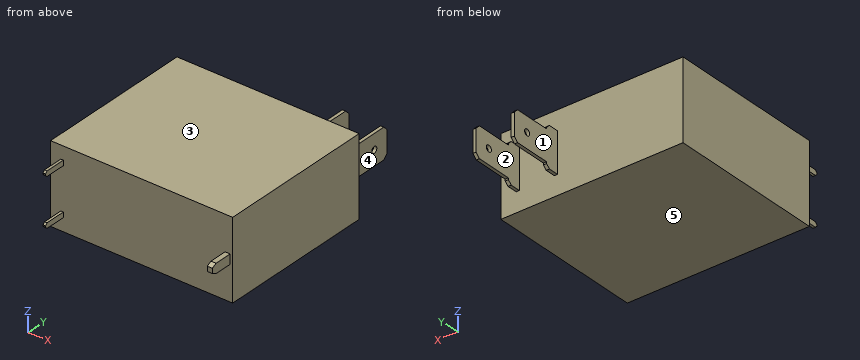
from build123d import *

# Parameters (mm, degrees)
CROQUIS1_W              = 28.6
CROQUIS1_H              = 12.4
SALIENTE_EXTRUIR1_DEPTH = 24.9
CROQUIS2_R              = 0.5
SALIENTE_EXTRUIR2_DEPTH = 0.25
SALIENTE_EXTRUIR3_DEPTH = 0.4
SALIENTE_EXTRUIR4_DEPTH = 0.2


with BuildPart() as part:
    # Croquis1 → Saliente-Extruir1 (new body)
    with BuildSketch(Plane(origin=(0, 0, 0), x_dir=(1, 0, 0), z_dir=(0, 1, 0))):
        with Locations((14.3, 6.2)):
            Rectangle(CROQUIS1_W, CROQUIS1_H)
    extrude(amount=SALIENTE_EXTRUIR1_DEPTH)

    # Croquis2 → Saliente-Extruir2 (add, symmetric)
    with BuildSketch(Plane(origin=(25.95, 0, 0), x_dir=(0, 0, -1), z_dir=(1, 0, 0))):
        Polygon((3.05, 24.9), (3.05, 26.504259841), (3.5733005, 27.05), (3.825, 27.05), (3.825, 32.761976859), (4.463023141, 33.4), (7.936976859, 33.4), (8.575, 32.761976859), (8.575, 27.05), (8.8266995, 27.05), (9.35, 26.504259841), (9.35, 24.9), align=None)
        with Locations((6.2, 30.9)):
            Circle(CROQUIS2_R, mode=Mode.SUBTRACT)
    saliente_extruir2 = extrude(amount=SALIENTE_EXTRUIR2_DEPTH, both=True)

    # Simetría1: Saliente-Extruir2 across plane
    add(saliente_extruir2.mirror(Plane(origin=(22.95, 0, 0), x_dir=(0, 0, 1), z_dir=(1, 0, 0))))

    # Croquis4 → Saliente-Extruir3 (add, symmetric)
    with BuildSketch(Plane.ZY.offset(-27.8)):
        Polygon((-6.95, 0), (-6.95, -2.77742352), (-6.577466383, -3.5), (-5.822533617, -3.5), (-5.45, -2.77742352), (-5.45, 0), align=None)
    extrude(amount=SALIENTE_EXTRUIR3_DEPTH, both=True)

    # Croquis6 → Saliente-Extruir4 (add, symmetric)
    with BuildSketch(Plane.ZY.offset(-1.8)):
        Polygon((-10.35, 0), (-10.35, -3.200399192), (-10.050399192, -3.5), (-9.849600808, -3.5), (-9.55, -3.200399192), (-9.55, 0), align=None)
        Polygon((-2.85, 0), (-2.05, 0), (-2.05, -3.200399192), (-2.349600808, -3.5), (-2.550399192, -3.5), (-2.85, -3.200399192), align=None)
    extrude(amount=SALIENTE_EXTRUIR4_DEPTH, both=True)


solid = part.part
Here's how the part is built. I have some questions about the finished solid (model axes, mm). Face numbers are marked on the shaded views. A direction names the side the tool comes from. Coordinates: 2 decimals unless noted, no trailing zeros. Order: outer loops, then holes, each group sorted by start corner. A loop starts at its lowest first (then second) coordinate and runs counter-clockwise, first axis right, second up.
Item 1: If we section it at A-A on y = 30.9: List the corners of the cut face in (x, z) for me (3 decimals), plus the area to 3 significant figures.
Result sheet:
outline: (19.7, -8.575) - (20.2, -8.575) - (20.2, -6.7) - (19.7, -6.7) - close; (19.7, -5.7) - (20.2, -5.7) - (20.2, -3.825) - (19.7, -3.825) - close; (25.7, -8.575) - (26.2, -8.575) - (26.2, -6.7) - (25.7, -6.7) - close; (25.7, -5.7) - (26.2, -5.7) - (26.2, -3.825) - (25.7, -3.825) - close
area: 3.75 mm2
Item 2: For P1, Ø2, axis at y = 26.5, z = -9, coming from the -X side; P2, Ø4, axis at x = 9, z = -3.5, coming from the +Y side; P3, Ø0.6, axis at x = 26, y = 25.5, coming from the +Z side, each with a flat end and sliding along its axis, tell me the tip position at first contact or that it passes through.
Result sheet:
P1: stops at x = 19.7
P2: stops at y = 24.9
P3: stops at z = -3.05
Item 3: For the marked faces 4 and 5, which set-ups out of +Z, -Z, +X, -X, +Y, -Y let a thin tool reach every point of the face, with its end or its side?
Result sheet:
face 4: +Z, -Z, +X, +Y
face 5: -Z, +X, -X, +Y, -Y
Item 4: If we section it at B-B on x = 4.5: List the corners of the cut face in (y, z) for me.
Result sheet:
outline: (0, -12.4) - (24.9, -12.4) - (24.9, 0) - (0, 0) - close
Item 5: If we mould it in two halves opening along X, with no side actions, what happens to the marked faces 1, 2 and 3? For each: +X half, -X half, draft (parallel to the pull), parting line (faces both ways), or undercut.
Result sheet:
face 1: -X half
face 2: undercut
face 3: draft
Item 6: I need wall thicknesses on line 1 (X direction, y = 26, z = -5); line 2 (Y direction, x = 20, z = -6.2); line 3 (Y direction, x = 5, z = -6.5). Which ranges of each line are inside material? Lowest first, please.
Result sheet:
line 1: x = 19.7 to 20.2, 25.7 to 26.2
line 2: y = 0 to 30.4, 31.4 to 33.4
line 3: y = 0 to 24.9
